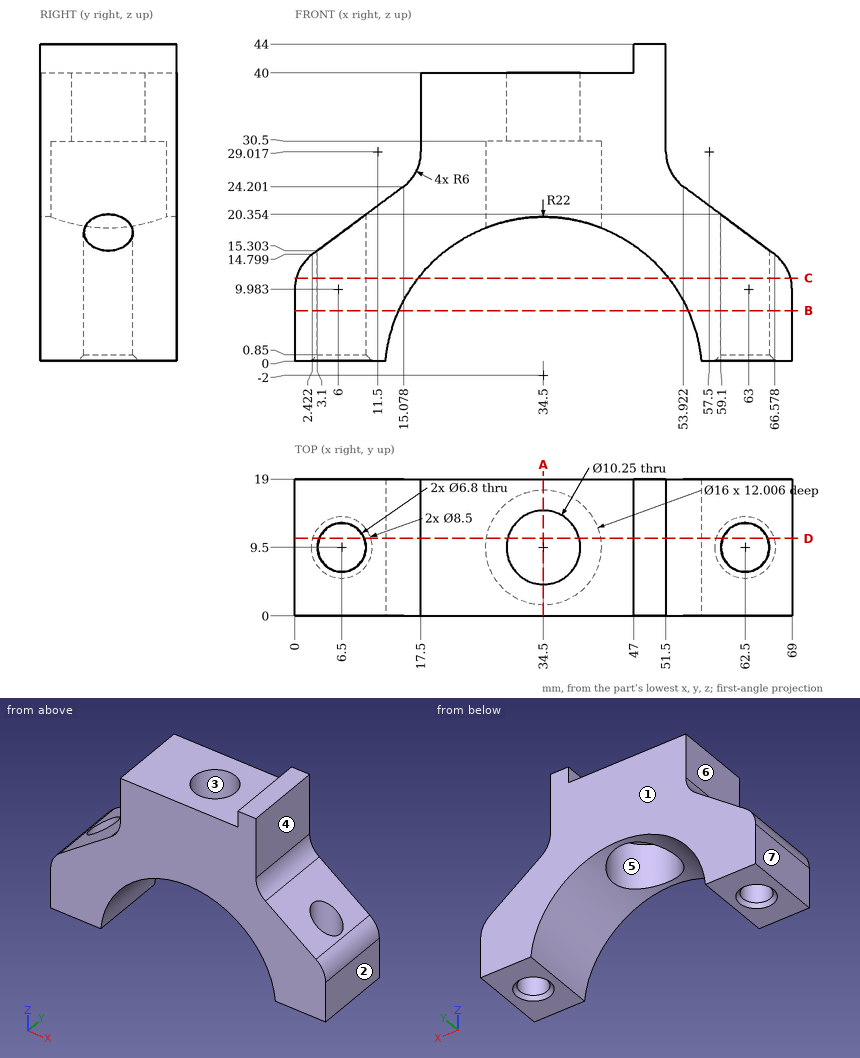
Answer from the drawing. Dimensions are ordinates in mm from the lowest x, y and z of the part. A direction names the side the tool comes from. Round coordinates to 2 decimals unless told otherwise and drop trailing zeros. Loops run counter-clockwise (first coordinate to the right, second up) from the corner with the lowest first, then second, coordinate; pieces in that order, holes last.
1) For the marked faces 4, 5, 6 and 7, determine the directions among +Z, -Z, +X, -X, +Y, -Y from which every point of the face is accessible in a straight line to the end or side of a thin tool.
Outcome:
face 4: +Z, +X, +Y, -Y
face 5: -Z
face 6: +Z, -X, +Y, -Y
face 7: +Z, -Z, -X, +Y, -Y
2) Consider line 1 (Y direction, x = 34.5, z = 35.75) (1 decimal); line 2 (X direction, y = 11.5, z = 10); line 3 (Z direction, x = 30, y = 3.5). Determine where each line is inside the solid, lowest interval first.
Outcome:
line 1: y = 0 to 4.4, 14.6 to 19
line 2: x = 0 to 3.75, 9.25 to 16.06, 52.94 to 59.75, 65.25 to 69
line 3: z = 30.5 to 40
3) Given P1, Ø7.5, axis at y = 5, z = 34, coming from the +X side; P2, Ø8, axis at x = 23.5, y = 5.5, coming from the +Z side; P3, Ø3, axis at y = 7, z = 41, coming from the -X side, each flat-ended and moving along its own axis, determine where each tip first touches the part or whether it passes through.
Outcome:
P1: stops at x = 51.5
P2: stops at z = 40
P3: stops at x = 17.5
4) A cutting plane is placed at C-C on z = 11.5. Determine the outline of the cut face in (x, y) (1 decimal), plus the area to 3 significant figures.
Outcome:
outline: (0.2, 0) - (17.1, 0) - (17.1, 19) - (0.2, 19) - close; (51.9, 0) - (68.8, 0) - (68.8, 19) - (51.9, 19) - close; hole circle Ø6.8 at (6.5, 9.5); hole circle Ø6.8 at (62.5, 9.5)
area: 571 mm2
5) A cutting plane is placed at D-D on y = 10.75. Give the number of separate pieces and of enclosed holes in the cut face, plus the area to 3 significant figures.
Outcome:
separate pieces: 4
enclosed holes: 0
area: 893 mm2
6) For a pull along Y with two mould halves and no side action, classify the marked faces 1, 2 and 3 as released by +Y, released by -Y, zero draft, split by the parting line, or undercut.
Outcome:
face 1: released by +Y
face 2: zero draft
face 3: undercut
7) A cutting plane is placed at B-B on z = 7. Determine the outline of the cut face in (x, y) (1 decimal).
Outcome:
outline: (0, 0) - (14.4, 0) - (14.4, 19) - (0, 19) - close; (54.6, 0) - (69, 0) - (69, 19) - (54.6, 19) - close; hole circle Ø6.8 at (6.5, 9.5); hole circle Ø6.8 at (62.5, 9.5)
8) A cutting plane is placed at A-A on x = 34.5. Determine the outline of the cut face in (y, z) (1 decimal).
Outcome:
outline: (0, 20) - (1.5, 20) - (1.5, 30.5) - (4.4, 30.5) - (4.4, 40) - (0, 40) - close; (14.6, 30.5) - (17.5, 30.5) - (17.5, 20) - (19, 20) - (19, 40) - (14.6, 40) - close
